```python
from build123d import *

# Parameters (mm, degrees)
SKETCH_1_W      = 370
SKETCH_1_H      = 370
SKETCH_1_W_2    = 350
SKETCH_1_H_2    = 350
EXTRUDE_1_DEPTH = 50
SKETCH_2_W      = 370
SKETCH_2_H      = 370
EXTRUDE_2_DEPTH = 200
SKETCH_3_W      = 350
SKETCH_3_H      = 350
SKETCH_3_W_2    = 250
SKETCH_3_H_2    = 250
EXTRUDE_3_DEPTH = 1


with BuildPart() as part:
    # 草图1 → 凸台-拉伸1 (new body)
    with BuildSketch(Plane(origin=(0, 0, 0), x_dir=(1, 0, 0), z_dir=(0, 1, 0))):
        Rectangle(SKETCH_1_W, SKETCH_1_H)
        Rectangle(SKETCH_1_W_2, SKETCH_1_H_2, mode=Mode.SUBTRACT)
    extrude(amount=EXTRUDE_1_DEPTH)

    # 草图2 → 凸台-拉伸2 (add)
    with BuildSketch(Plane.XZ):
        Rectangle(SKETCH_2_W, SKETCH_2_H)
    extrude(amount=EXTRUDE_2_DEPTH)

    # 草图3 → 凸台-拉伸3 (add)
    with BuildSketch(Plane(origin=(0, 0, 0), x_dir=(1, 0, 0), z_dir=(0, 1, 0))):
        Rectangle(SKETCH_3_W, SKETCH_3_H)
        Rectangle(SKETCH_3_W_2, SKETCH_3_H_2, mode=Mode.SUBTRACT)
    extrude(amount=EXTRUDE_3_DEPTH)


solid = part.part
```
Here's how the part is built. I have some questions about the finished solid (model axes, mm). A direction names the side the tool comes from. Coordinates: 2 decimals unless noted, no trailing zeros. Order: outer loops, then holes, each group sorted by start corner. A loop starts at its lowest first (then second) coordinate and runs counter-clockwise, first axis right, second up. Notation, with made-up numbers: (29.5, 80) - (49.5, 80) arc R32 ccw to (49.5, 110) - close; hole circle Ø3 at (46.25, 65). An arc over 180 degrees is marked (long way). One line per question, with ' | ' between items. Start each with the question number.
1. If we section it at A-A (z = -159): Write out the boundary of the cut face in (x, y).
2. If we section it at D-D (z = 59): Write out the boundary of the cut face in (x, y).
3. Which directions (+Z, -Z, +X, -X, +Y, -Y) give clear straight access to the entire face, cutting with the end or side of a thin tool? Please do faces 1 (the flat face through (-3, -73, -185)), 2 (the flat face through (-2, 25, -175)).
4. If we section it at B-B (x = 17): Write out the boundary of the cut face in (y, z), and give its area (3 significant figures).
5. I'm going to push a flat-ended pin straight in: pin 1 Ø10 at (x, z) = (-6.5, -25.5) entering from +Y. Where does the tip first touch, or does it pass through?
6. Please list where these lines run through material, in increasing order: line 1 along X through (y, z) = (5, -17.5); line 2 along Y through (x, z) = (48.5, -47). Write a range as [from, to].
7. If we section it at C-C (y = 33): Write out the boundary of the cut face in (x, z).
Model answer:
1) outline: (-185, -200) - (185, -200) - (185, 50) - (175, 50) - (175, 1) - (-175, 1) - (-175, 50) - (-185, 50) - close
2) outline: (-185, -200) - (185, -200) - (185, 50) - (175, 50) - (175, 1) - (125, 1) - (125, 0) - (-125, 0) - (-125, 1) - (-175, 1) - (-175, 50) - (-185, 50) - close
3) face 1: -Z, +X, -X, +Y, -Y | face 2: +Y
4) outline: (-200, -185) - (50, -185) - (50, -175) - (1, -175) - (1, -125) - (0, -125) - (0, 125) - (1, 125) - (1, 175) - (50, 175) - (50, 185) - (-200, 185) - close | area: 75,100 mm²
5) pin 1: stops at y = 0
6) line 1: x = [-185, -175], [175, 185] | line 2: y = [-200, 0]
7) outline: (-185, -185) - (185, -185) - (185, 185) - (-185, 185) - close; hole (-175, -175) - (175, -175) - (175, 175) - (-175, 175) - close
